Check sheet for the modelled part. Datum: model origin and axes. Units: mm. A direction names the side the tool comes from. Give positions to 0.01 mm unless a question says otherwise; leave off trailing zeros. Order: outer loops, then holes, each group sorted by start corner. A loop starts at its lowest first (then second) coordinate and runs counter-clockwise, first axis right, second up.
Item 1: Material ranges on line 1 along Y through (x, z) = (30, 0.75); line 2 along Y through (x, z) = (30, 3.8); line 3 along Y through (x, z) = (-19.4, 1.65), recorded low to high.
Item 2: Access from +Z, -Z, +X, -X, +Y, -Y to the whole of each face (thin tool, end or side, straight path). Record for faces 1 (the flat face through (-20, 18, 6)), 2 (the cylindrical face through (-15.154, 27.187, 2.465)), 3 (the cylindrical face through (25.83, 24.31, 4.01)).
Item 3: Sectioned sample at D-D on x = 23. Record the boundary of the cut face in (y, z), and give its area (3 significant figures).
Item 4: Sectioned sample at B-B on z = 6.5. Record the boundary of the cut face in (x, y), and give its area (3 significant figures).
Item 5: Sectioned sample at A-A on x = -19.4. Record the boundary of the cut face in (y, z).
Item 6: Sectioned sample at C-C on x = -29.5. Record the boundary of the cut face in (y, z), and give its area (3 significant figures).
Item 7: Gauge pin test, flat ends, axial feed: P1, Ø1.5, axis at x = -12.5, z = 7, coming from the +Y side; P2, Ø8, axis at x = -30, y = -27.5, coming from the +Z side; P3, Ø3, axis at x = -13, y = -8, coming from the +Z side. Record the tip position at first contact, or that the pin passes through.
from build123d import *

# Parameters (mm, degrees)
F0_W            = 72.8
F0_H            = 69
F1_DEPTH        = 5
F3_D            = 7
F5_D            = 8.5
F6_W            = 34
F6_H            = 36
F6_W_2          = 31
F6_H_2          = 31
F7_DEPTH        = 3
F9_D            = 9
F9_CSINK_D      = 18
F9_CSINK_ANGLE  = 90
F11_D           = 7
F11_CBORE_D     = 10.5
F11_CBORE_DEPTH = 2


with BuildPart() as f1:
    # F0 (on Top) → F1 (new body)
    with BuildSketch(Plane.XY):
        Rectangle(F0_W, F0_H)
    extrude(amount=F1_DEPTH)

    # F3 (through all)
    with Locations(Plane.XY.offset(5)):
        with Locations((-30, 27.5), (30, 27.5), (30, -27.5), (-30, -27.5)):
            Hole(F3_D / 2)

    # F5 (through all)
    with Locations(Plane.XY.offset(5)):
        with Locations((-19.4, 27), (-19.4, -28)):
            Hole(F5_D / 2)

    # F6 (on face) → F7 (join)
    with BuildSketch(Plane.XY.offset(5)):
        with Locations((-19.4, 0)):
            Rectangle(F6_W, F6_H)
        with Locations((-19.4, 0)):
            Rectangle(F6_W_2, F6_H_2, mode=Mode.SUBTRACT)
    extrude(amount=F7_DEPTH)

    # F9 (through all)
    with Locations(Plane(origin=(0, 0, 0), x_dir=(1, 0, 0), z_dir=(0, 0, -1))):
        with Locations((-19.4, 0)):
            CounterSinkHole(F9_D / 2, F9_CSINK_D / 2, counter_sink_angle=F9_CSINK_ANGLE)

    # F11 (through all)
    with Locations(Plane.XY.offset(5)):
        with Locations((-30, 27.5), (30, 27.5), (30, -27.5), (-30, -27.5)):
            CounterBoreHole(F11_D / 2, F11_CBORE_D / 2, F11_CBORE_DEPTH)


solid = f1.part
Report:
1. line 1: y = -34.5 to -31, -24 to 24, 31 to 34.5
1. line 2: y = -34.5 to -32.75, -22.25 to 22.25, 32.75 to 34.5
1. line 3: y = -34.5 to -32.25, -23.75 to -7.35, 7.35 to 22.75, 31.25 to 34.5
2. face 1: +Z, +X, -X, +Y
2. face 2: +Z, -Z
2. face 3: +Z
3. outline: (-34.5, 0) - (34.5, 0) - (34.5, 5) - (-34.5, 5) - close
3. area: 345 mm2
4. outline: (-36.4, -18) - (-2.4, -18) - (-2.4, 18) - (-36.4, 18) - close; hole (-34.9, -15.5) - (-3.9, -15.5) - (-3.9, 15.5) - (-34.9, 15.5) - close
4. area: 263 mm2
5. outline: (-34.5, 0) - (-32.25, 0) - (-32.25, 5) - (-34.5, 5) - close; (-23.75, 0) - (-9, 0) - (-4.5, 4.5) - (-4.5, 5) - (-15.5, 5) - (-15.5, 8) - (-18, 8) - (-18, 5) - (-23.75, 5) - close; (4.5, 4.5) - (9, 0) - (22.75, 0) - (22.75, 5) - (18, 5) - (18, 8) - (15.5, 8) - (15.5, 5) - (4.5, 5) - close; (31.25, 0) - (34.5, 0) - (34.5, 5) - (31.25, 5) - close
6. outline: (-34.5, 0) - (-30.96, 0) - (-30.96, 3) - (-32.73, 3) - (-32.73, 5) - (-34.5, 5) - close; (-24.04, 0) - (24.04, 0) - (24.04, 3) - (22.27, 3) - (22.27, 5) - (18, 5) - (18, 8) - (15.5, 8) - (15.5, 5) - (-15.5, 5) - (-15.5, 8) - (-18, 8) - (-18, 5) - (-22.27, 5) - (-22.27, 3) - (-24.04, 3) - close; (30.96, 0) - (34.5, 0) - (34.5, 5) - (32.73, 5) - (32.73, 3) - (30.96, 3) - close
6. area: 277 mm2
7. P1: stops at y = 18
7. P2: stops at z = 3
7. P3: stops at z = 5
